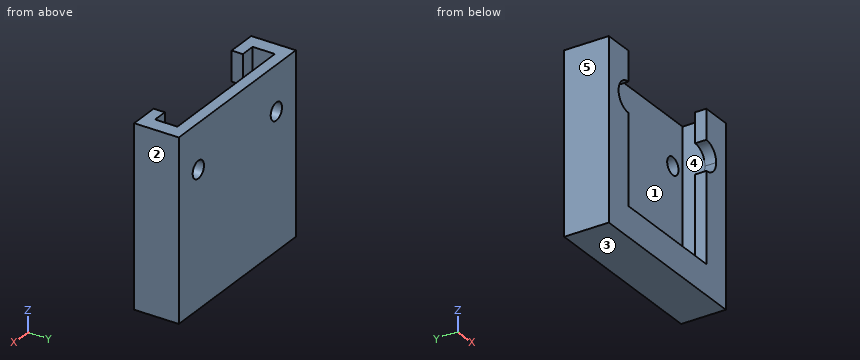
from build123d import *

# Parameters (mm, degrees)
F1_DEPTH = 19.05
F2_W     = 6.35
F2_H     = 4.7625
F2_W_2   = 50.8
F3_DEPTH = 63.5
F5_DEPTH = 10.16
F8_DEPTH = 12.7


with BuildPart() as f1:
    # F0 (on Front) → F1 (new body)
    with BuildSketch(Plane.XZ):
        Polygon((0, -38.1), (0, 0), (0, 38.1), (-38.1, 38.1), (-38.1, 0), (-38.1, -38.1), align=None)
        Polygon((0, 38.1), (0, 0), (0, -38.1), (38.1, -38.1), (38.1, 0), (38.1, 38.1), align=None)
    extrude(amount=F1_DEPTH)

    # F2 (on face) → F3 (cut)
    with BuildSketch(Plane.XY.offset(38.1)):
        Polygon((-25.4, -14.2875), (25.4, -14.2875), (25.4, -9.525), (25.4, -4.7625), (-25.4, -4.7625), (-25.4, -9.525), align=None)
        with Locations((28.575, -11.90625)):
            Rectangle(F2_W, F2_H)
        with Locations((28.575, -7.14375)):
            Rectangle(F2_W, F2_H)
        with Locations((-28.575, -11.90625)):
            Rectangle(F2_W, F2_H)
        with Locations((-28.575, -7.14375)):
            Rectangle(F2_W, F2_H)
        with Locations((0, -16.66875)):
            Rectangle(F2_W_2, F2_H)
    extrude(amount=-F3_DEPTH, mode=Mode.SUBTRACT)

    # F4 (on face) → F5 (cut)
    with BuildSketch(Plane(origin=(0, 0, 0), x_dir=(-1, 0, 0), z_dir=(0, 1, 0))):
        with BuildLine():
            ThreePointArc((-29.083, 19.05), (-25.4, 15.367), (-21.717, 19.05))
            Line((-21.717, 19.05), (-25.4, 19.05))
            Line((-25.4, 19.05), (-29.083, 19.05))
        make_face()
        with BuildLine():
            Line((-25.4, 19.05), (-21.717, 19.05))
            ThreePointArc((-21.717, 19.05), (-25.4, 22.733), (-29.083, 19.05))
            Line((-29.083, 19.05), (-25.4, 19.05))
        make_face()
        with BuildLine():
            ThreePointArc((29.083, 19.05), (25.4, 22.733), (21.717, 19.05))
            Line((21.717, 19.05), (25.4, 19.05))
            Line((25.4, 19.05), (29.083, 19.05))
        make_face()
        with BuildLine():
            Line((25.4, 19.05), (21.717, 19.05))
            ThreePointArc((21.717, 19.05), (25.4, 15.367), (29.083, 19.05))
            Line((29.083, 19.05), (25.4, 19.05))
        make_face()
    extrude(amount=-F5_DEPTH, mode=Mode.SUBTRACT)

    # F7 (on face) → F8 (cut)
    with BuildSketch(Plane.XZ.offset(19.05)):
        with BuildLine():
            ThreePointArc((-25.4, 25.3892062068), (-29.8901280605, 14.5490781463), (-19.05, 19.0392062068))
            ThreePointArc((-19.05, 19.0392062068), (-20.9098719395, 23.5293342673), (-25.4, 25.3892062068))
        make_face()
        with BuildLine():
            ThreePointArc((25.4, 25.4), (20.9098719395, 14.5598719395), (31.75, 19.05))
            ThreePointArc((31.75, 19.05), (29.8901280605, 23.5401280605), (25.4, 25.4))
        make_face()
    extrude(amount=-F8_DEPTH, mode=Mode.SUBTRACT)


solid = f1.part
Model file for the job. Use its own axes, mm. Face numbers are marked on the shaded views. A direction names the side the tool comes from. Round coordinates to 2 decimals unless told otherwise and drop trailing zeros. Order: outer loops, then holes, each group sorted by start corner. A loop starts at its lowest first (then second) coordinate and runs counter-clockwise, first axis right, second up.
(1) Drill centre lines: line 1 (Z direction, x = -25.4, y = -2.9); line 2 (X direction, y = -8.75, z = 1); line 3 (Y direction, x = -24.5, z = -22). Where is each one in solid material? Low to high.
(2) 3-axis set-ups, long thin cutter, end or side, ignore diameter. For the marked faces 1 and 2: which of +Z, -Z, +X, -X, +Y, -Y reach the whole face in a straight line?
(3) Pin check, flat tips, straight feed: pin 1 (1.5 mm diameter, centred on x = 8.5, z = -5.5, fed in from -Y); pin 2 (3 mm diameter, centred on x = -27.5, z = -10, fed in from +Y). Stop position of each tip, or through.
(4) Band-saw the part on C-C (z = -16). List the corners of the cut face in (x, y), then the cut area to 3 significant figures.
(5) Band-saw the part on D-D (y = -16.75). List the corners of the cut face in (x, z), then the cut area to 3 significant figures.
(6) Band-saw the part on B-B (x = 24). List the corners of the cut face in (y, z), then the cut area to 3 significant figures.
(7) Pull direction X, two halves, no side cores. Call the marked faces 3, 4 and 5: released by +X, released by -X, zero draft, split by the parting line, or undercut.
(8) Band-saw the part on A-A (y = -11.25). List the corners of the cut face in (x, z).
Verdict:
1. line 1: z = -38.1 to 15.37, 22.73 to 38.1
1. line 2: x = -38.1 to -31.75, 31.75 to 38.1
1. line 3: y = -4.76 to 0
2. face 1: +Z
2. face 2: +Z, -Z, +X, +Y, -Y
3. pin 1: stops at y = -4.76
3. pin 2: stops at y = 0
4. outline: (-38.1, -19.05) - (-25.4, -19.05) - (-25.4, -14.29) - (-31.75, -14.29) - (-31.75, -4.76) - (31.75, -4.76) - (31.75, -14.29) - (25.4, -14.29) - (25.4, -19.05) - (38.1, -19.05) - (38.1, 0) - (-38.1, 0) - close
4. area: 605 mm2
5. outline: (-38.1, -38.1) - (38.1, -38.1) - (38.1, 38.1) - (25.4, 38.1) - (25.4, 25.4) arc R6.35 cw to (25.4, 12.7) - (25.4, -25.4) - (-25.4, -25.4) - (-25.4, 12.69) arc R6.35 cw to (-25.4, 25.39) - (-25.4, 38.1) - (-38.1, 38.1) - close
5. area: 2,450 mm2
6. outline: (-19.05, -38.1) - (0, -38.1) - (0, 15.64) - (-4.76, 15.64) - (-4.76, -25.4) - (-19.05, -25.4) - close; (-4.76, 22.46) - (0, 22.46) - (0, 38.1) - (-4.76, 38.1) - close
6. area: 512 mm2
7. face 3: zero draft
7. face 4: undercut
7. face 5: released by -X
8. outline: (-38.1, -38.1) - (38.1, -38.1) - (38.1, 38.1) - (31.75, 38.1) - (31.75, -25.4) - (-31.75, -25.4) - (-31.75, 38.1) - (-38.1, 38.1) - close
